Part model, mm, in its own coordinate system. Face numbers are marked on the shaded views. A direction names the side the tool comes from. Give positions to 0.01 mm unless a question says otherwise; leave off trailing zeros. Loops run counter-clockwise (first coordinate to the right, second up) from the corner with the lowest first, then second, coordinate; pieces in that order, holes last. Notation, with made-up numbers: (45, 25) -> (96, 25) arc R16 ccw to (96, 51) -> close; hole circle Ø4 at (55.5, -34.5). An arc over 180 degrees is marked (long way). One line per question, with ' | ' between items.
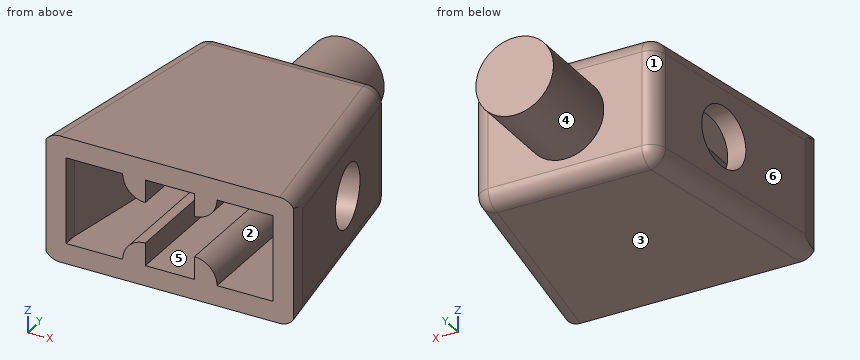
```python
from build123d import *

# Parameters (mm, degrees)
BOSS_EXTRUDE1_DEPTH = 3.9
SHELL5_T            = -1.25
SKETCH2_R           = 2.4
BOSS_EXTRUDE2_DEPTH = 5.5
BOSS_EXTRUDE3_DEPTH = 12.45
SKETCH6_R           = 0.7
CUT_EXTRUDE2_DEPTH  = 4.25
CUT_EXTRUDE3_REACH  = 17.264
SKETCH7_R           = 1.9
CUT_EXTRUDE4_REACH  = 17.264
SKETCH8_R           = 1.9
FILLET1_R           = 1


with BuildPart() as part:
    # Sketch1 → Boss-Extrude1 (new body, symmetric)
    with BuildSketch(Plane.XY):
        Polygon((-7.65, -5.85), (-7.65, -6.85), (7.65, -6.85), (7.65, -5.85), (5.599872407, 6.85), (-5.600127593, 6.85), align=None)
    extrude(amount=BOSS_EXTRUDE1_DEPTH, both=True)

    # Shell5
    shell5_openings = [part.faces().sort_by_distance(p)[0] for p in [
        (0, -6.85, 0),
    ]]
    offset(amount=SHELL5_T, openings=shell5_openings, kind=Kind.INTERSECTION)

    # Sketch2 → Boss-Extrude2 (add)
    with BuildSketch(Plane(origin=(0, 6.85, 0), x_dir=(1, 0, 0), z_dir=(0, 1, 0))):
        Circle(SKETCH2_R)
    extrude(amount=BOSS_EXTRUDE2_DEPTH)

    # Sketch5 → Boss-Extrude3 (add, through all)
    with BuildSketch(Plane.XZ.offset(-5.6)):
        with BuildLine():
            Line((-1.5, 1.25), (-1.5, 2.65))
            Line((-1.5, 2.65), (-2.9, 2.65))
            ThreePointArc((-2.9, 2.65), (-2.489949494, 1.660050506), (-1.5, 1.25))
        make_face()
        with BuildLine():
            Line((1.530768156, 2.65), (1.530768156, 1.25))
            ThreePointArc((1.530768156, 1.25), (2.52071765, 1.660050506), (2.930768156, 2.65))
            Line((2.930768156, 2.65), (1.530768156, 2.65))
        make_face()
        with BuildLine():
            Line((-1.5, -1.25), (-1.5, -2.65))
            Line((-1.5, -2.65), (-2.9, -2.65))
            ThreePointArc((-2.9, -2.65), (-2.489949494, -1.660050506), (-1.5, -1.25))
        make_face()
        with BuildLine():
            Line((1.530768156, -2.65), (1.530768156, -1.25))
            ThreePointArc((1.530768156, -1.25), (2.52071765, -1.660050506), (2.930768156, -2.65))
            Line((2.930768156, -2.65), (1.530768156, -2.65))
        make_face()
    extrude(amount=BOSS_EXTRUDE3_DEPTH)

    # Sketch6 → Cut-Extrude2 (cut)
    with BuildSketch(Plane.XZ.offset(-5.6)):
        Circle(SKETCH6_R)
    extrude(amount=-CUT_EXTRUDE2_DEPTH, mode=Mode.SUBTRACT)

    # Sketch7 → Cut-Extrude3 (cut, up to next)
    with BuildSketch(Plane(origin=(6.535346626, 1.054983815, 0), x_dir=(0, 0, -1), z_dir=(0.987219843, 0.159364302, 0)), mode=Mode.PRIVATE) as cut_extrude3_sk1:
        Circle(SKETCH7_R)
    cut_extrude3_tool1 = extrude(cut_extrude3_sk1.sketch, amount=-CUT_EXTRUDE3_REACH, mode=Mode.PRIVATE) & part.part
    add(cut_extrude3_tool1.solids().sort_by_distance((6.535347, 1.054984, 0))[0], mode=Mode.SUBTRACT)

    # Sketch8 → Cut-Extrude4 (cut, up to next)
    with BuildSketch(Plane(origin=(-6.535502505, 1.054877658, 0), x_dir=(0, 0, 1), z_dir=(-0.987222964, 0.15934497, 0)), mode=Mode.PRIVATE) as cut_extrude4_sk1:
        Circle(SKETCH8_R)
    cut_extrude4_tool1 = extrude(cut_extrude4_sk1.sketch, amount=-CUT_EXTRUDE4_REACH, mode=Mode.PRIVATE) & part.part
    add(cut_extrude4_tool1.solids().sort_by_distance((-6.535503, 1.054878, 0))[0], mode=Mode.SUBTRACT)

    # Fillet1
    fillet1_edges = [part.edges().sort_by_distance(p)[0] for p in [
        (-6.625063797, 0.5, -3.9),
        (6.624936203, 0.5, -3.9),
        (-0.000127593, 6.85, -3.9),
        (-5.600127593, 6.85, 0),
        (-6.625063797, 0.5, 3.9),
        (-0.000127593, 6.85, 3.9),
        (6.624936203, 0.5, 3.9),
        (5.599872407, 6.85, 0),
    ]]
    fillet(fillet1_edges, radius=FILLET1_R)


solid = part.part
```
1) Saw through at A-A (z = 1.5). State how many separate pieces and enclosed holes the cut face has, and give its area (3 significant figures).
Found:
separate pieces: 3 | enclosed holes: 0 | area: 80.1 mm2
2) Saw through at D-D (x = 0). Give the cut face in (y, z), and give its area (3 significant figures).
Found:
outline: (-6.85, -3.9) -> (5.85, -3.9) arc R1 ccw to (6.85, -2.9) -> (6.85, -2.4) -> (12.35, -2.4) -> (12.35, 2.4) -> (6.85, 2.4) -> (6.85, 2.9) arc R1 ccw to (5.85, 3.9) -> (-6.85, 3.9) -> (-6.85, 2.65) -> (5.6, 2.65) -> (5.6, 0.7) -> (9.85, 0.7) -> (9.85, -0.7) -> (5.6, -0.7) -> (5.6, -2.65) -> (-6.85, -2.65) -> close | area: 60.9 mm2
3) Saw through at B-B (x = -3.5). Give the cut face in (y, z), and give its area (3 significant figures).
Found:
outline: (-6.85, -3.9) -> (5.85, -3.9) arc R1 ccw to (6.85, -2.9) -> (6.85, 2.9) arc R1 ccw to (5.85, 3.9) -> (-6.85, 3.9) -> (-6.85, 2.65) -> (5.6, 2.65) -> (5.6, -2.65) -> (-6.85, -2.65) -> close | area: 40.4 mm2
4) Pull direction Z, two halves, no side cores. Call the marked faces 1, 2 and 3: pulls with the +Z half, pulls with the -Z half, needs draft (parallel to the pull), parting line crosses it, or undercut.
Found:
face 1: needs draft | face 2: undercut | face 3: pulls with the -Z half
5) Pin check, flat tips, straight feed: P1, Ø0.7, axis at y = 1.5, z = 2, coming from the +X side; P2, Ø1.1, axis at x = 0, z = -0.5, coming from the -Y side; P3, Ø1.1, axis at y = -1, z = -2, coming from the +X side. Stop position of each tip, or through.
Found:
P1: x = 6.52 | P2: y = 5.6 | P3: x = 6.96
6) Saw through at C-C (y = 7.5). Give the cut face in (x, z).
Found:
outline: circle Ø4.8 at (0, 0); hole circle Ø1.4 at (0, 0)
7) Tool access for the marked faces 4, 5 and 6: list every direction of +Z, -Z, +X, -X, +Y, -Y with a clear straight run to the whole face (end or side of a thin tool).
Found:
face 4: +Y | face 5: -Y | face 6: +Z, -Z, -X, +Y
8) Drill centre lines: line 1 (Z direction, x = 0, y = 8.9); line 2 (Z direction, x = -4.75, y = -4.75); line 3 (Y direction, x = -3.75, z = 1). Where is each one in solid material? Low to high.
Found:
line 1: -2.4 to -0.7, 0.7 to 2.4 | line 2: -3.9 to -2.65, 2.65 to 3.9 | line 3: 5.6 to 6.85
